```python
from build123d import *

# Parameters (mm, degrees)
EXTRUDE_1_DEPTH     = 4
SKETCH_2_R          = 1.6
CUT_EXTRUDE_1_DEPTH = 68.670041634
SKETCH_3_R          = 6
EXTRUDE_2_DEPTH     = 6


with BuildPart() as part:
    # 草图1 → 凸台-拉伸1 (new body)
    with BuildSketch(Plane.XY):
        Polygon((58.413097366, -10.348521791), (52.263097366, -10.348521791), (52.263097366, -6.928521791), (24.563097366, -6.928521791), (24.563097366, -10.348521791), (18.413097366, -10.348521791), (18.413097366, -30.508521791), (24.563097366, -30.508521791), (24.563097366, -33.928521791), (52.263097366, -33.928521791), (52.263097366, -30.508521791), (58.413097366, -30.508521791), align=None)
    extrude(amount=EXTRUDE_1_DEPTH)

    # 草图2 → 切除-拉伸1 (cut, through all)
    with BuildSketch(Plane.XY.offset(4)):
        with Locations((32.413097366, -20.428521791)):
            Circle(SKETCH_2_R)
    extrude(amount=-CUT_EXTRUDE_1_DEPTH, mode=Mode.SUBTRACT)

    # 草图3 → 凸台-拉伸2 (add)
    with BuildSketch(Plane.XY.offset(4)):
        with Locations((32.413097366, -20.428521791)):
            Circle(SKETCH_3_R)
        Polygon((33.971943092, -23.128521791), (35.530788819, -20.428521791), (33.971943092, -17.728521791), (30.854251639, -17.728521791), (29.295405912, -20.428521791), (30.854251639, -23.128521791), align=None, mode=Mode.SUBTRACT)
    extrude(amount=EXTRUDE_2_DEPTH)


solid = part.part
```
Check sheet for the modelled part. Datum: model origin and axes. Units: mm. A direction names the side the tool comes from. Give positions to 0.01 mm unless a question says otherwise; leave off trailing zeros. Write each loop counter-clockwise with the first axis right and the second up, starting at its lowest first coordinate (ties: lowest second). Pieces come first, ordered by that corner, then holes. Notation, with made-up numbers: (11.25, -3.75) - (31.25, -3.75) arc R25 cw to (31.25, 28.25) - close; hole circle Ø9 at (-32.5, -37). An arc over 180 degrees is marked (long way). Answer as a JSON object with one key per item and string values. Group by question number.
1) Thickness scan on probe 1 along Z at (x, y) = (37, -27.75); probe 2 along X at (y, z) = (-22.75, 4.5); probe 3 along Y at (x, z) = (24.5, 3). Record the ranges inside material, lowest first. Write a range as from..to.
2) Depth check by flat-ended pin: P1, Ø1.2, axis at x = 55, z = 2.5, coming from the +Y side; P2, Ø3, axis at x = 22.5, z = 1.5, coming from the -Y side; P3, Ø1, axis at y = -33, z = 1.5, coming from the +X side. Enter the tip coordinate at first touch or a pass-through.
3) Sectioned sample at B-B (y = -20). Record the cut outline in (x, z), then the cut area to 3 significant figures.
4) Sectioned sample at C-C (x = 27.5). Record the cut outline in (y, z).
5) Sectioned sample at D-D (y = -26). Record the cut outline in (x, z).
6) Access from +Z, -Z, +X, -X, +Y, -Y to the whole of each face (thin tool, end or side, straight path). Record for faces 1 (the face through (30.086, -19.06, 6.958)), 2 (the face through (52.263, -32, 2)), 3 (the face through (22, -10.349, 2)), 4 (the face through (21, -30.509, 2)), 5 (the face through (55, -10.349, 2)).
7) Release check for a two-part mould opening along Y. For faces 6 (the face through (27.65, -24.08, 6.96)), 7 (the face through (34.762, -19.097, 6.958)), 8 (the face through (58.413, -21, 2)) record: pulls with the +Y half, pulls with the -Y half, needs draft (parallel to the pull), parting line crosses it, or undercut.
8) Sectioned sample at A-A (z = 1.25). Record the cut outline in (x, y).
Geometry results:
{
 "1": {"probe 1": "z = 0..4", "probe 2": "x = 26.88..30.64, 34.19..37.95", "probe 3": "y = -30.51..-10.35"},
 "2": {"P1": "stops at y = -10.35", "P2": "stops at y = -30.51", "P3": "stops at x = 52.26"},
 "3": {"outline": "(18.41, 0) - (30.87, 0) - (30.87, 4) - (29.54, 4) - (29.54, 10) - (26.43, 10) - (26.43, 4) - (18.41, 4) - close; (33.95, 0) - (58.41, 0) - (58.41, 4) - (38.4, 4) - (38.4, 10) - (35.28, 10) - (35.28, 4) - (33.95, 4) - close", "area": "185 mm^2"},
 "4": {"outline": "(-33.93, 0) - (-6.93, 0) - (-6.93, 4) - (-16.98, 4) - (-16.98, 10) - (-23.87, 10) - (-23.87, 4) - (-33.93, 4) - close"},
 "5": {"outline": "(18.41, 0) - (58.41, 0) - (58.41, 4) - (34.64, 4) - (34.64, 10) - (30.19, 10) - (30.19, 4) - (18.41, 4) - close"},
 "6": {"face 1": "+Z", "face 2": "+Z, -Z, +X, -Y", "face 3": "+Z, -Z, -X, +Y", "face 4": "+Z, -Z, -X, -Y", "face 5": "+Z, -Z, +X, +Y"},
 "7": {"face 6": "parting line crosses it", "face 7": "undercut", "face 8": "needs draft"},
 "8": {"outline": "(18.41, -30.51) - (24.56, -30.51) - (24.56, -33.93) - (52.26, -33.93) - (52.26, -30.51) - (58.41, -30.51) - (58.41, -10.35) - (52.26, -10.35) - (52.26, -6.93) - (24.56, -6.93) - (24.56, -10.35) - (18.41, -10.35) - close; hole circle Ø3.2 at (32.41, -20.43)"}
}
